from build123d import *

# Parameters (mm, degrees)
Y_KSEKLIK_EKSTR_ZYON1_DEPTH = 10
SKETCH3_R                   = 1.5
CUT_EXTRUDE1_DEPTH          = 10


with BuildPart() as part:
    # Çizim1 → Yükseklik-Ekstrüzyon1 (new body)
    with BuildSketch(Plane(origin=(0, 0, 0), x_dir=(0, 0, -1), z_dir=(1, 0, 0))):
        Polygon((0, 0), (260, 0), (260, 167.95), (60, 167.95), (0, 107.95), align=None)
    extrude(amount=Y_KSEKLIK_EKSTR_ZYON1_DEPTH)

    # Sketch3 → Cut-Extrude1 (cut)
    with BuildSketch(Plane(origin=(10, 0, 0), x_dir=(0, 0, -1), z_dir=(1, 0, 0))):
        with Locations((130, 83.975)):
            Circle(SKETCH3_R)
    extrude(amount=-CUT_EXTRUDE1_DEPTH, mode=Mode.SUBTRACT)


solid = part.part
Geometry check sheet. Reference: the model listing, model coordinates, mm. Give positions to 0.01 mm unless a question says otherwise; leave off trailing zeros. Order: outer loops, then holes, each group sorted by start corner. A loop starts at its lowest first (then second) coordinate and runs counter-clockwise, first axis right, second up. Notation, with made-up numbers: (-13.5, -39) - (-6.5, -39) arc R17 cw to (-6.5, -32) - close; hole circle Ø9 at (-37.75, 88). An arc over 180 degrees is marked (long way). Use one line per item in the form item = value.
1) Sectioned sample at B-B (x = 5.75). Record the boundary of the cut face in (y, z) (3 decimals), and give its area (3 significant figures).
Working result:
outline = (0, -260) - (167.95, -260) - (167.95, -60) - (107.95, 0) - (0, 0) - close; hole circle Ø3 at (83.975, -130)
area = 41,900 mm^2
2) Depth check by flat-ended pin: pin 1 Ø2.5 at (y, z) = (83.975, -130) entering from +X. Enter the tip coordinate at first touch or a pass-through.
Working result:
pin_1 = through
3) Sectioned sample at A-A (y = 157). Record the boundary of the cut face in (x, z).
Working result:
outline = (0, -260) - (10, -260) - (10, -49.05) - (0, -49.05) - close
4) Material ranges on probe 1 along Y at (x, z) = (5, -130) (3 decimals); probe 2 along Y at (x, z) = (8.5, -29.5); probe 3 along Y at (x, z) = (8.5, -42.5), recorded low to high. Write a range as from..to.
Working result:
probe_1 = 0..82.475, 85.475..167.95
probe_2 = 0..137.45
probe_3 = 0..150.45
